```python
from build123d import *

# Parameters (mm, degrees)
SKETCH_1_W               = 250
SKETCH_1_H               = 115
SKETCH_1_R               = 3.5
SKETCH_1_R_2             = 1.55
EXTRUDE_1_DEPTH          = 4
SKETCH_2_R               = 45
SKETCH_2_R_2             = 32.5
CUT_EXTRUDE_1_DEPTH      = 2
SKETCH_3_R               = 10.05
SKETCH_3_R_2             = 1.7
CUT_EXTRUDE_2_DEPTH      = 1
CUT_EXTRUDE_5_DEPTH      = 20
CUT_EXTRUDE_5_DEPTH_BACK = 20
SKETCH_4_R               = 1.7
FILLET_1_R               = 10


with BuildPart() as part:
    # 草图1 → 凸台-拉伸1 (new body)
    with BuildSketch(Plane(origin=(0, 0, 0), x_dir=(1, 0, 0), z_dir=(0, 1, 0))):
        Rectangle(SKETCH_1_W, SKETCH_1_H)
        with Locations(Location((0, 0, 0), (0, 0, 270))):
            Circle(SKETCH_1_R, mode=Mode.SUBTRACT)
        with Locations(Location((45, 49, 0), (0, 0, 270))):
            Circle(SKETCH_1_R_2, mode=Mode.SUBTRACT)
        with Locations(Location((45, -49, 0), (0, 0, 90))):
            Circle(SKETCH_1_R_2, mode=Mode.SUBTRACT)
        with Locations(Location((-45, -49, 0), (0, 0, 270))):
            Circle(SKETCH_1_R_2, mode=Mode.SUBTRACT)
        with Locations(Location((-45, 49, 0), (0, 0, 90))):
            Circle(SKETCH_1_R_2, mode=Mode.SUBTRACT)
        with Locations(Location((-15, -49, 0), (0, 0, 270))):
            Circle(SKETCH_1_R_2, mode=Mode.SUBTRACT)
        with Locations(Location((15, -49, 0), (0, 0, 90))):
            Circle(SKETCH_1_R_2, mode=Mode.SUBTRACT)
        with Locations(Location((15, 49, 0), (0, 0, 270))):
            Circle(SKETCH_1_R_2, mode=Mode.SUBTRACT)
        with Locations(Location((-15, 49, 0), (0, 0, 90))):
            Circle(SKETCH_1_R_2, mode=Mode.SUBTRACT)
        with Locations(Location((30, 49, 0), (0, 0, 270))):
            Circle(SKETCH_1_R_2, mode=Mode.SUBTRACT)
        with Locations(Location((-30, 49, 0), (0, 0, 270))):
            Circle(SKETCH_1_R_2, mode=Mode.SUBTRACT)
        with Locations(Location((-30, -49, 0), (0, 0, 270))):
            Circle(SKETCH_1_R_2, mode=Mode.SUBTRACT)
        with Locations(Location((30, -49, 0), (0, 0, 270))):
            Circle(SKETCH_1_R_2, mode=Mode.SUBTRACT)
    extrude(amount=EXTRUDE_1_DEPTH)

    # 草图2 → 切除-拉伸1 (cut)
    with BuildSketch(Plane(origin=(0, 4, 0), x_dir=(1, 0, 0), z_dir=(0, 1, 0))):
        with Locations(Location((0, 0, 0), (0, 0, 270))):
            Circle(SKETCH_2_R)
        with Locations(Location((0, 0, 0), (0, 0, 270))):
            Circle(SKETCH_2_R_2, mode=Mode.SUBTRACT)
    extrude(amount=-CUT_EXTRUDE_1_DEPTH, mode=Mode.SUBTRACT)

    # 草图3 → 切除-拉伸2 (cut)
    with BuildSketch(Plane(origin=(0, 4, 0), x_dir=(1, 0, 0), z_dir=(0, 1, 0))):
        with Locations(Location((0, 0, 0), (0, 0, 270))):
            Circle(SKETCH_3_R)
        with Locations(Location((0, 7, 0), (0, 0, 270))):
            Circle(SKETCH_3_R_2, mode=Mode.SUBTRACT)
        with Locations(Location((7, 0, 0), (0, 0, 270))):
            Circle(SKETCH_3_R_2, mode=Mode.SUBTRACT)
        with Locations(Location((0, -7, 0), (0, 0, 270))):
            Circle(SKETCH_3_R_2, mode=Mode.SUBTRACT)
        with Locations(Location((-7, 0, 0), (0, 0, 270))):
            Circle(SKETCH_3_R_2, mode=Mode.SUBTRACT)
    extrude(amount=-CUT_EXTRUDE_2_DEPTH, mode=Mode.SUBTRACT)

    # 草图4 → 切除-拉伸5 (cut, two sides: drawn at the far end of the back side and taken through both)
    with BuildSketch(Plane(origin=(0, 3, 0), x_dir=(1, 0, 0), z_dir=(0, 1, 0)).offset(-CUT_EXTRUDE_5_DEPTH_BACK)):
        with Locations(Location((7, 0, 0), (0, 0, 90))):
            Circle(SKETCH_4_R)
        with Locations(Location((0, 7, 0), (0, 0, 90))):
            Circle(SKETCH_4_R)
        with Locations(Location((0, -7, 0), (0, 0, 90))):
            Circle(SKETCH_4_R)
        with Locations(Location((-7, 0, 0), (0, 0, 90))):
            Circle(SKETCH_4_R)
    extrude(amount=CUT_EXTRUDE_5_DEPTH + CUT_EXTRUDE_5_DEPTH_BACK, mode=Mode.SUBTRACT)

    # 圆角1
    fillet_1_edges = [part.edges().sort_by_distance(p)[0] for p in [
        (125, 2, 57.5),
        (-125, 2, 57.5),
        (-125, 2, -57.5),
        (125, 2, -57.5),
    ]]
    fillet(fillet_1_edges, radius=FILLET_1_R)


solid = part.part
```
The listing builds one solid part. Answer for the finished solid, in the listing's coordinates (mm). A direction names the side the tool comes from. Give positions to 0.01 mm unless a question says otherwise; leave off trailing zeros. Write each loop counter-clockwise with the first axis right and the second up, starting at its lowest first coordinate (ties: lowest second). Pieces come first, ordered by that corner, then holes. Notation, with made-up numbers: (54, -29) -> (94, -29) arc R18 cw to (94, -13) -> close; hole circle Ø8 at (-23, -17.75). An arc over 180 degrees is marked (long way). Use one line per item in the form item = value.
1) Straight lines are drawn through the part: probe 1 along X at (y, z) = (0.85, 0); probe 2 along X at (y, z) = (2.4, 8); probe 3 along X at (y, z) = (2.7, 0.5). For each, find the intervals that lie inside material, in ascending order.
Result:
probe_1 = -125 to -8.7, -5.3 to -3.5, 3.5 to 5.3, 8.7 to 125
probe_2 = -125 to -44.28, -31.5 to -1.37, 1.37 to 31.5, 44.28 to 125
probe_3 = -125 to -45, -32.5 to -8.62, -5.38 to -3.46, 3.46 to 5.38, 8.62 to 32.5, 45 to 125
2) This flat-tipped pin is pushed along its axis until it touches: P1, Ø4.5, axis at x = -7, z = 0, coming from the +Y side. Where does it stop, or does it pass through?
Result:
P1 = 3
3) Section A-A on x = 40 is taken. Write down the section's boundary in (y, z), plus the area to 3 significant figures.
Result:
outline = (0, -57.5) -> (4, -57.5) -> (4, -20.62) -> (2, -20.62) -> (2, 20.62) -> (4, 20.62) -> (4, 57.5) -> (0, 57.5) -> close
area = 378 mm²
4) A tool of negligible diameter and unlimited length cuts with its end or side. For faces 4 (the flat face through (7, 4, -8)), 5 (the cylindrical face through (0.44, 3.51, -10.04)), from which of +Z, -Z, +X, -X, +Y, -Y can it reach the whole face along a straight path? Write none if from no direction.
Result:
face_4 = +Z, -Z, +X, -X, +Y
face_5 = +Y
5) Section B-B on x = -38 is taken. Write down the section's boundary in (y, z).
Result:
outline = (0, -57.5) -> (4, -57.5) -> (4, -24.1) -> (2, -24.1) -> (2, 24.1) -> (4, 24.1) -> (4, 57.5) -> (0, 57.5) -> close
6) For a pull along Z with two mould halves and no side action, classify faces 1 (the flat face through (26, 4, -39)), 2 (the cylindrical face through (-122.15, 2.03, -54.49)), 3 (the flat face through (0, 3, 4)) as +Z half, -Z half, draft (parallel to the pull), parting line (faces both ways), or undercut.
Result:
face_1 = draft
face_2 = -Z half
face_3 = undercut
